Input: part model. Units: mm. Frame: model coordinates. A direction names the side the tool comes from. Give positions to 0.01 mm unless a question says otherwise; leave off trailing zeros. Loops run counter-clockwise (first coordinate to the right, second up) from the corner with the lowest first, then second, coordinate; pieces in that order, holes last. Notation, with made-up numbers: (56, 40.25) -> (64, 40.25) arc R4 ccw to (64, 46.25) -> close; hole circle Ø10 at (28.5, 15.5). An arc over 180 degrees is marked (long way). Use CSV: the item, a comma, the result in double quotes.
```python
from build123d import *

# Parameters (mm, degrees)
SKETCH1_W           = 299.030753262
SKETCH1_H           = 176
BOSS_EXTRUDE1_DEPTH = 28.765376631
SKETCH2_W           = 297.030753262
SKETCH2_H           = 27.765376631
CUT_EXTRUDE1_DEPTH  = 372.704572948
SKETCH3_W           = 29
SKETCH3_H           = 47
CUT_EXTRUDE2_DEPTH  = 366.805713875
SKETCH4_W           = 134.5
SKETCH4_H           = 1
BOSS_EXTRUDE2_DEPTH = 55.265376631
SKETCH5_W           = 134.5
SKETCH5_H           = 1
BOSS_EXTRUDE3_DEPTH = 151.265376631
SKETCH6_W           = 128
SKETCH6_H           = 1
BOSS_EXTRUDE4_DEPTH = 55.265376631
SKETCH7_W           = 128
SKETCH7_H           = 1
BOSS_EXTRUDE5_DEPTH = 151.265376631
SKETCH8_W           = 289.5
SKETCH8_H           = 1
BOSS_EXTRUDE6_DEPTH = 3.765376631
SKETCH9_W           = 289.5
SKETCH9_H           = 1
BOSS_EXTRUDE7_DEPTH = 27.765376631
SKETCH10_W          = 57.5
SKETCH10_H          = 148
CUT_EXTRUDE3_DEPTH  = 430.032610708
SKETCH11_W          = 58
SKETCH11_H          = 148
CUT_EXTRUDE4_DEPTH  = 430.032610708
FILLET1_R           = 0.7366
FILLET2_R           = 1
FILLET3_R           = 1.7366


with BuildPart() as part:
    # Sketch1 → Boss-Extrude1 (new body)
    with BuildSketch(Plane(origin=(0, 0, -1), x_dir=(-1, 0, 0), z_dir=(0, 0, -1))):
        with Locations((176.701381692, -75)):
            Rectangle(SKETCH1_W, SKETCH1_H)
    extrude(amount=-BOSS_EXTRUDE1_DEPTH)

    # Sketch2 → Cut-Extrude1 (cut, through all)
    with BuildSketch(Plane.XZ.offset(163)):
        with Locations((-176.701381692, 13.882688316)):
            Rectangle(SKETCH2_W, SKETCH2_H)
    extrude(amount=-CUT_EXTRUDE1_DEPTH, mode=Mode.SUBTRACT)

    # Sketch3 → Cut-Extrude2 (cut, through all)
    with BuildSketch(Plane(origin=(0, 0, -1), x_dir=(-1, 0, 0), z_dir=(0, 0, -1))):
        with Locations((173.451381692, -10.5)):
            Rectangle(SKETCH3_W, SKETCH3_H)
    extrude(amount=-CUT_EXTRUDE2_DEPTH, mode=Mode.SUBTRACT)

    # Sketch4 → Boss-Extrude2 (add)
    with BuildSketch(Plane(origin=(0, 13, 0), x_dir=(-1, 0, 0), z_dir=(0, 1, 0))):
        with Locations((255.201381692, -0.5)):
            Rectangle(SKETCH4_W, SKETCH4_H)
    extrude(amount=BOSS_EXTRUDE2_DEPTH)

    # Sketch5 → Boss-Extrude3 (add)
    with BuildSketch(Plane.XY):
        with Locations((-255.201381692, 67.765376631)):
            Rectangle(SKETCH5_W, SKETCH5_H)
    extrude(amount=BOSS_EXTRUDE3_DEPTH)

    # Sketch6 → Boss-Extrude4 (add)
    with BuildSketch(Plane(origin=(0, 13, 0), x_dir=(-1, 0, 0), z_dir=(0, 1, 0))):
        with Locations((94.951381692, -0.5)):
            Rectangle(SKETCH6_W, SKETCH6_H)
    extrude(amount=BOSS_EXTRUDE4_DEPTH)

    # Sketch7 → Boss-Extrude5 (add)
    with BuildSketch(Plane.XY):
        with Locations((-94.951381692, 67.765376631)):
            Rectangle(SKETCH7_W, SKETCH7_H)
    extrude(amount=BOSS_EXTRUDE5_DEPTH)

    # Sketch8 → Boss-Extrude6 (add)
    with BuildSketch(Plane.XZ.offset(163)):
        with Locations((-176.701381692, -0.5)):
            Rectangle(SKETCH8_W, SKETCH8_H)
    extrude(amount=BOSS_EXTRUDE6_DEPTH)

    # Sketch9 → Boss-Extrude7 (add)
    with BuildSketch(Plane.XY):
        with Locations((-176.701381692, -166.265376631)):
            Rectangle(SKETCH9_W, SKETCH9_H)
    extrude(amount=BOSS_EXTRUDE7_DEPTH)

    # Sketch10 → Cut-Extrude3 (cut, through all)
    with BuildSketch(Plane.XZ.offset(-67.265376631)):
        with Locations((-293.701381692, 77.265376631)):
            Rectangle(SKETCH10_W, SKETCH10_H)
    extrude(amount=-CUT_EXTRUDE3_DEPTH, mode=Mode.SUBTRACT)

    # Sketch11 → Cut-Extrude4 (cut, through all)
    with BuildSketch(Plane.XZ.offset(-67.265376631)):
        with Locations((-59.951381692, 77.265376631)):
            Rectangle(SKETCH11_W, SKETCH11_H)
    extrude(amount=-CUT_EXTRUDE4_DEPTH, mode=Mode.SUBTRACT)

    # Fillet1
    fillet1_edges = [part.edges().sort_by_distance(p)[0] for p in [
        (-176.701381692, -165.765376631, 0),
        (-28.186005061, -75, 0),
        (-325.216758323, -75, 0),
        (-255.201381692, 67.265376631, 0),
        (-94.951381692, 67.265376631, 0),
    ]]
    fillet(fillet1_edges, radius=FILLET1_R)

    # Fillet2
    fillet2_edges = [part.edges().sort_by_distance(p)[0] for p in [
        (-325.716758323, 13, 27.765376631),
        (-321.451381692, -166.265376631, 27.765376631),
        (-31.951381692, -166.265376631, 27.765376631),
        (-264.951381692, 67.765376631, 151.265376631),
        (-325.716758323, -163, 27.765376631),
        (-27.686005061, 13, 27.765376631),
        (-88.951381692, 67.765376631, 151.265376631),
        (-27.686005061, -163, 27.765376631),
        (-187.951381692, 67.765376631, 151.265376631),
        (-158.951381692, 67.765376631, 151.265376631),
    ]]
    fillet(fillet2_edges, radius=FILLET2_R)

    # Fillet3
    fillet3_edges = [part.edges().sort_by_distance(p)[0] for p in [
        (-176.701381692, -166.765376631, -1),
        (-27.186005061, -75, -1),
        (-255.201381692, 68.265376631, -1),
        (-326.216758323, -75, -1),
        (-94.951381692, 68.265376631, -1),
    ]]
    fillet(fillet3_edges, radius=FILLET3_R)


solid = part.part
```
1) Section query D-D (z = 22.5). Return loops of the section in (x, y).
From the geometry:
outline,"(-326.22, -163) -> (-325.22, -163) -> (-325.22, 13) -> (-326.22, 13) -> close; (-321.45, -166.77) -> (-31.95, -166.77) -> (-31.95, -165.77) -> (-321.45, -165.77) -> close; (-264.95, 67.27) -> (-187.95, 67.27) -> (-187.95, 68.27) -> (-264.95, 68.27) -> close; (-158.95, 67.27) -> (-88.95, 67.27) -> (-88.95, 68.27) -> (-158.95, 68.27) -> close; (-28.19, -163) -> (-27.19, -163) -> (-27.19, 13) -> (-28.19, 13) -> close"
2) Contact query for flat-ended pins moving along their axis: pin 1 (1.1 mm diameter, centred on x = -27.5, y = -31.5, fed in from +Z); pin 2 (1 mm diameter, centred on x = -167.5, y = -97, fed in from +Z); pin 3 (4 mm diameter, centred on x = -325, z = 18.5, fed in from +Y). Output: stop coordinate, or through.
From the geometry:
pin 1,"stops at z = 27.77"
pin 2,"stops at z = 0"
pin 3,"stops at y = 13"
3) Section query A-A (z = 74). Return loops of the section in (x, y), then the cut area to 3 significant figures.
From the geometry:
outline,"(-264.95, 67.27) -> (-187.95, 67.27) -> (-187.95, 68.27) -> (-264.95, 68.27) -> close; (-158.95, 67.27) -> (-88.95, 67.27) -> (-88.95, 68.27) -> (-158.95, 68.27) -> close"
area,"147 mm^2"
4) Ray query, line 1 (X direction, y = -110.5, z = 14); line 2 (Z direction, x = -139, y = -87); line 3 (Y direction, x = -120.5, z = 51). Return the intervals inside material, ascending.
From the geometry:
line 1,"x = -326.22 to -325.22, -28.19 to -27.19"
line 2,"z = -1 to 0"
line 3,"y = 67.27 to 68.27"
5) Section query B-B (y = 28.5). Return loops of the section in (x, z), then the cut area to 4 significant figures.
From the geometry:
outline,"(-322.45, -1) -> (-187.95, -1) -> (-187.95, 0) -> (-322.45, 0) -> close; (-158.95, -1) -> (-30.95, -1) -> (-30.95, 0) -> (-158.95, 0) -> close"
area,"262.5 mm^2"
6) Section query C-C (y = -49). Return loops of the section in (x, z).
From the geometry:
outline,"(-326.22, 0.74) arc R1.74 ccw to (-324.48, -1) -> (-28.92, -1) arc R1.74 ccw to (-27.19, 0.74) -> (-27.19, 27.77) -> (-28.19, 27.77) -> (-28.19, 0.74) arc R0.74 cw to (-28.92, 0) -> (-324.48, 0) arc R0.74 cw to (-325.22, 0.74) -> (-325.22, 27.77) -> (-326.22, 27.77) -> close"
7) Mould query, pull axis X, two halves, no side actions, for faces 1 (the flat face through (-325.217, -76, 14)), 2 (the flat face through (-27.186, -76, 14)), 3 (the flat face through (-226, 67.265, 75)), 4 (the flat face through (-28.186, -76, 14)). Classes: pulls with the +X half, pulls with the -X half, needs draft (parallel to the pull), parting line crosses it, or undercut.
From the geometry:
face 1,"undercut"
face 2,"pulls with the +X half"
face 3,"needs draft"
face 4,"undercut"
8) Reachability of faces 5 (the flat face through (-175, -51, -1)), 6 (the flat face through (-175, -51, 0)), 7 (the flat face through (-124, 67.265, 75)) from +Z, -Z, +X, -X, +Y, -Y: full face, straight path, thin tool, end or side. Return the list, or none.
From the geometry:
face 5,"-Z, +X, -X, +Y, -Y"
face 6,"+Z"
face 7,"+Z, +X, -X"
